Geometry check sheet. Reference: drawing and pictorial views, mm from the part's lowest x, y, z. A direction names the side the tool comes from. Coordinates: 2 decimals unless noted, no trailing zeros. Write each loop counter-clockwise with the first axis right and the second up, starting at its lowest first coordinate (ties: lowest second). Pieces come first, ordered by that corner, then holes. Notation, with made-up numbers: (6.5, 6.25) -> (34.5, 6.25) arc R8 ccw to (34.5, 16.25) -> close; hole circle Ø6 at (66, 67). An arc over 180 degrees is marked (long way). Answer in a Markdown table with one row per item.
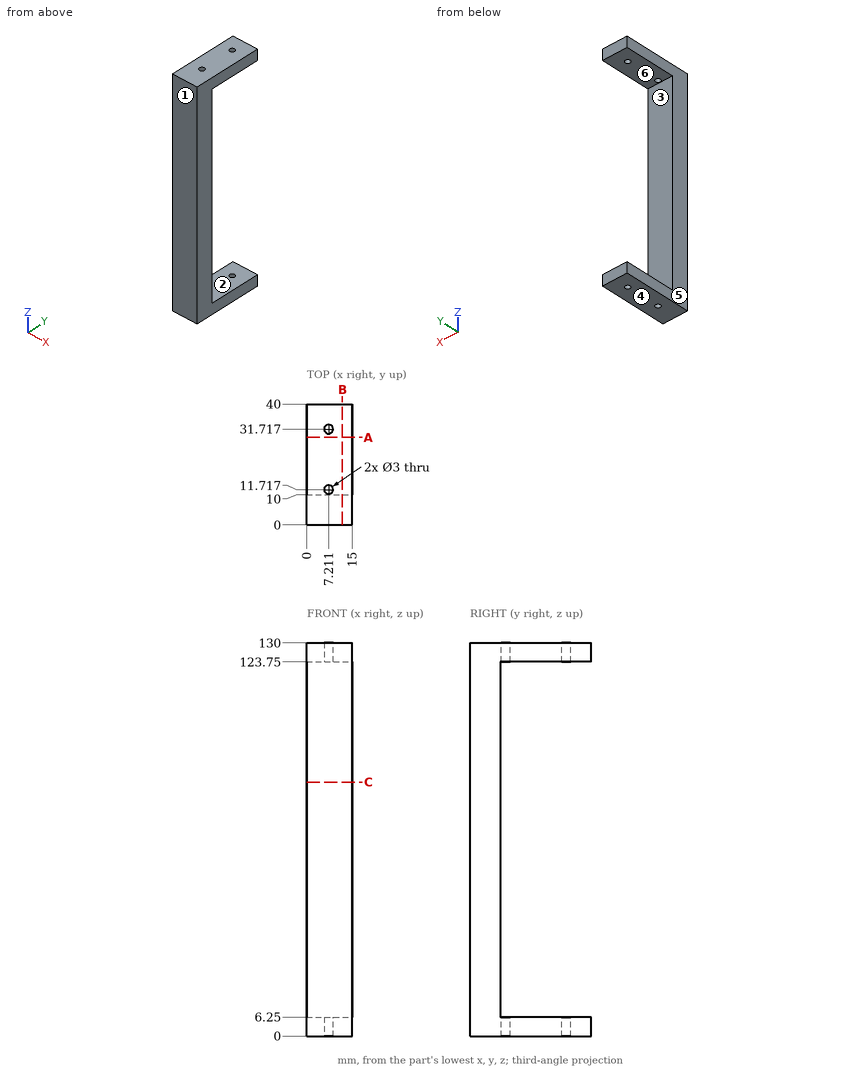
1. Thickness scan on line 1 (Z direction, x = 1, y = 28); line 2 (Y direction, x = 2.25, z = 110.5). Record the ranges inside material, lowest first. Write a range as from..to.
Geometry says:
| item | result |
|---|---|
| line 1 | 0..6.25, 123.75..130 |
| line 2 | 0..10 |
2. Section check B-B, the plane x = 11.75. Record the boundary of the cut face in (y, z), plus the area to 4 significant figures.
Geometry says:
| item | result |
|---|---|
| outline | (0, 0) -> (40, 0) -> (40, 6.25) -> (10, 6.25) -> (10, 123.75) -> (40, 123.75) -> (40, 130) -> (0, 130) -> close |
| area | 1,675 mm^2 |
3. Mould release check, pull along Z, two halves, no side actions. Record for the marked faces 1, 2, 3 and 4: released by +Z, released by -Z, zero draft, split by the parting line, or undercut.
Geometry says:
| item | result |
|---|---|
| face 1 | zero draft |
| face 2 | undercut |
| face 3 | undercut |
| face 4 | released by -Z |
4. Section check C-C, the plane z = 84. Record the boundary of the cut face in (x, y), plus the area to 3 significant figures.
Geometry says:
| item | result |
|---|---|
| outline | (0, 0) -> (15, 0) -> (15, 10) -> (0, 10) -> close |
| area | 150 mm^2 |
5. Section check A-A, the plane y = 29. Record the boundary of the cut face in (x, z).
Geometry says:
| item | result |
|---|---|
| outline | (0, 0) -> (15, 0) -> (15, 6.25) -> (0, 6.25) -> close; (0, 123.75) -> (15, 123.75) -> (15, 130) -> (0, 130) -> close |
6. Tool access check on the marked faces 5 and 6. Record the directions out of +Z, -Z, +X, -X, +Y, -Y that give a thin tool (end or side, any length) a straight path to the whole face; none if there is none.
Geometry says:
| item | result |
|---|---|
| face 5 | +Z, -Z, -X, +Y, -Y |
| face 6 | +X, -X, +Y |
